Design review of the part built by this model. Coordinates are the model's own, in mm. Round coordinates to 2 decimals unless told otherwise and drop trailing zeros. Loops run counter-clockwise (first coordinate to the right, second up) from the corner with the lowest first, then second, coordinate; pieces in that order, holes last. Notation, with made-up numbers: (19.5, 68) - (65.5, 68) arc R13 cw to (65.5, 74) - close; hole circle Ø5 at (38, 62.25). An arc over 180 degrees is marked (long way). Return JSON: item names as keys, results as strings. Group by question number.
(1) We need section C-C, the plane x = 0. Write out the cut boundary in (y, z), and give its area (3 significant figures).
(2) Wall thickness on L1, parallel to Y at x = -1, z = 0.6; L2, parallel to X at y = -99.75, z = 0.65; L3, parallel to X at y = 101.6, z = 0.5: over which ranges is each line inside the solid? List them lowest first. Write a range as [from, to].
(3) We need section D-D, the plane z = 0.25. Give the number of separate pieces and of enclosed holes in the cut face, and give its area (3 significant figures).
(4) We need section B-B, the plane y = -23.15. Write out the cut boundary in (x, z), and give its area (3 significant figures).
(5) We need section A-A, the plane x = 20.5. Write out the cut boundary in (y, z), and give its area (3 significant figures).
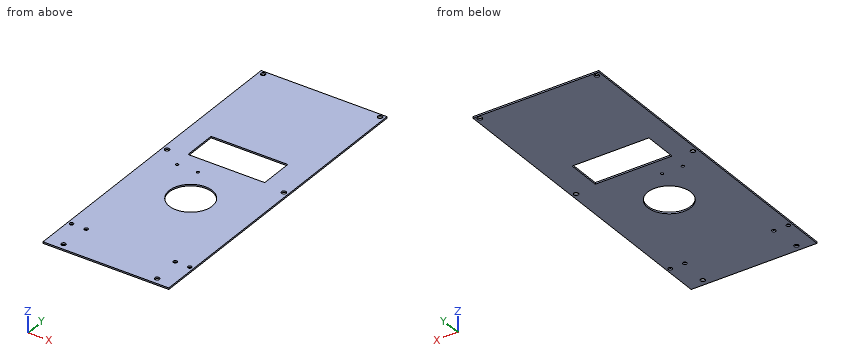
from build123d import *

# Parameters (mm, degrees)
SKETCH1_W                    = 82
SKETCH1_H                    = 208
BOSS_EXTRUDE1_DEPTH          = 1
F_3_0_3_DIAMETER_HOLE1_D     = 3
SKETCH8_R                    = 14
CUT_EXTRUDE1_DEPTH           = 10
SKETCH11_W                   = 50
SKETCH11_H                   = 22
CUT_EXTRUDE2_DEPTH           = 10
F_2_5_2_5_DIAMETER_HOLE1_D   = 2.5
F_1_75_1_75_DIAMETER_HOLE1_D = 1.75


with BuildPart() as part:
    # Sketch1 → Boss-Extrude1 (new body)
    with BuildSketch(Plane.XY):
        Rectangle(SKETCH1_W, SKETCH1_H)
    extrude(amount=BOSS_EXTRUDE1_DEPTH)

    # Ø3.0 (3) Diameter Hole1 (through all)
    with Locations(Plane.XY.offset(1)):
        with Locations((-38.1, 10), (38.1, 10), (30.5, -99.75), (-30.5, -99.75), (-38.1, 101.59999968), (38.1, 101.59999968)):
            Hole(F_3_0_3_DIAMETER_HOLE1_D / 2)

    # Sketch8 → Cut-Extrude1 (cut)
    with BuildSketch(Plane.XY.offset(1)):
        with Locations((0, -23.15)):
            Circle(SKETCH8_R)
    extrude(amount=-CUT_EXTRUDE1_DEPTH, mode=Mode.SUBTRACT)

    # Sketch11 → Cut-Extrude2 (cut)
    with BuildSketch(Plane.XY.offset(1)):
        with Locations((-1, 23.3)):
            Rectangle(SKETCH11_W, SKETCH11_H)
    extrude(amount=-CUT_EXTRUDE2_DEPTH, mode=Mode.SUBTRACT)

    # Ø2.5 (2.5) Diameter Hole1 (through all)
    with Locations(Plane.XY.offset(1)):
        with Locations((-38.5, -80.402796493), (-29, -80.402796493), (29, -80.402796493), (38.5, -80.402796493)):
            Hole(F_2_5_2_5_DIAMETER_HOLE1_D / 2)

    # Ø1.75 (1.75) Diameter Hole1 (through all)
    with Locations(Plane.XY.offset(1)):
        with Locations((-25.1, 0.65), (-11.6, 0.65)):
            Hole(F_1_75_1_75_DIAMETER_HOLE1_D / 2)


solid = part.part
Solutions:
{
 "1": {"outline": "(-104, 0) - (-37.15, 0) - (-37.15, 1) - (-104, 1) - close; (-9.15, 0) - (12.3, 0) - (12.3, 1) - (-9.15, 1) - close; (34.3, 0) - (104, 0) - (104, 1) - (34.3, 1) - close", "area": "158 mm^2"},
 "2": {"L1": "[-104, -37.11], [-9.19, 12.3], [34.3, 104]", "L2": "[-41, -32], [-29, 29], [32, 41]", "L3": "[-41, -39.6], [-36.6, 36.6], [39.6, 41]"},
 "3": {"separate pieces": "1", "enclosed holes": "14", "area": "15,300 mm^2"},
 "4": {"outline": "(-41, 0) - (-14, 0) - (-14, 1) - (-41, 1) - close; (14, 0) - (41, 0) - (41, 1) - (14, 1) - close", "area": "54.0 mm^2"},
 "5": {"outline": "(-104, 0) - (12.3, 0) - (12.3, 1) - (-104, 1) - close; (34.3, 0) - (104, 0) - (104, 1) - (34.3, 1) - close", "area": "186 mm^2"}
}
